Answer from the drawing. Dimensions are ordinates in mm from the lowest x, y and z of the part. A direction names the side the tool comes from. Round coordinates to 2 decimals unless told otherwise and drop trailing zeros. Write each loop counter-clockwise with the first axis right and the second up, starting at its lowest first coordinate (ties: lowest second). Pieces come first, ordered by that corner, then holes. Notation, with made-up numbers: (18, 69) -> (67, 69) arc R15 ccw to (67, 81) -> close; hole circle Ø7 at (-14, 81). An arc over 180 degrees is marked (long way). Return JSON: item names as keys, results as strings. Group by question number.
(1) For the marked faces 4 and 5, determine the directions among +Z, -Z, +X, -X, +Y, -Y from which every point of the face is accessible in a straight line to the end or side of a thin tool.
(2) Given pin 1 (2 mm diameter, centred on y = 4, z = 8.5, fed in from +X) (3 decimals); pin 2 (4 mm diameter, centred on x = 3.5, z = 8.5, fed in from +Y); pin 3 (1 mm diameter, centred on x = 3, z = 17.5, fed in from -Y), each flat-ended and moving along its own axis, determine where each tip first touches the part or whether it passes through.
(3) The mould has two halves that part along X. Classify the marked faces 1, 2 and 3: released by +X, released by -X, zero draft, split by the parting line, or undercut.
(4) A cutting plane is placed at D-D on z = 16.75. Give the vertices of the cut face in (x, y).
(5) A cutting plane is placed at B-B on y = 6.35. Give the vertices of the cut face in (x, z) (3 decimals).
(6) A cutting plane is placed at A-A on x = 6.35. Give the vertices of the cut face in (y, z) (3 decimals).
(7) A cutting plane is placed at C-C on x = 8.25. Give the vertices of the cut face in (y, z) (1 decimal).
(8) Straight lines are drawn through the part: line 1 (Y direction, x = 6.5, z = 9); line 2 (X direction, y = 1.5, z = 2.75). For each, find the intervals that lie inside material, in ascending order.
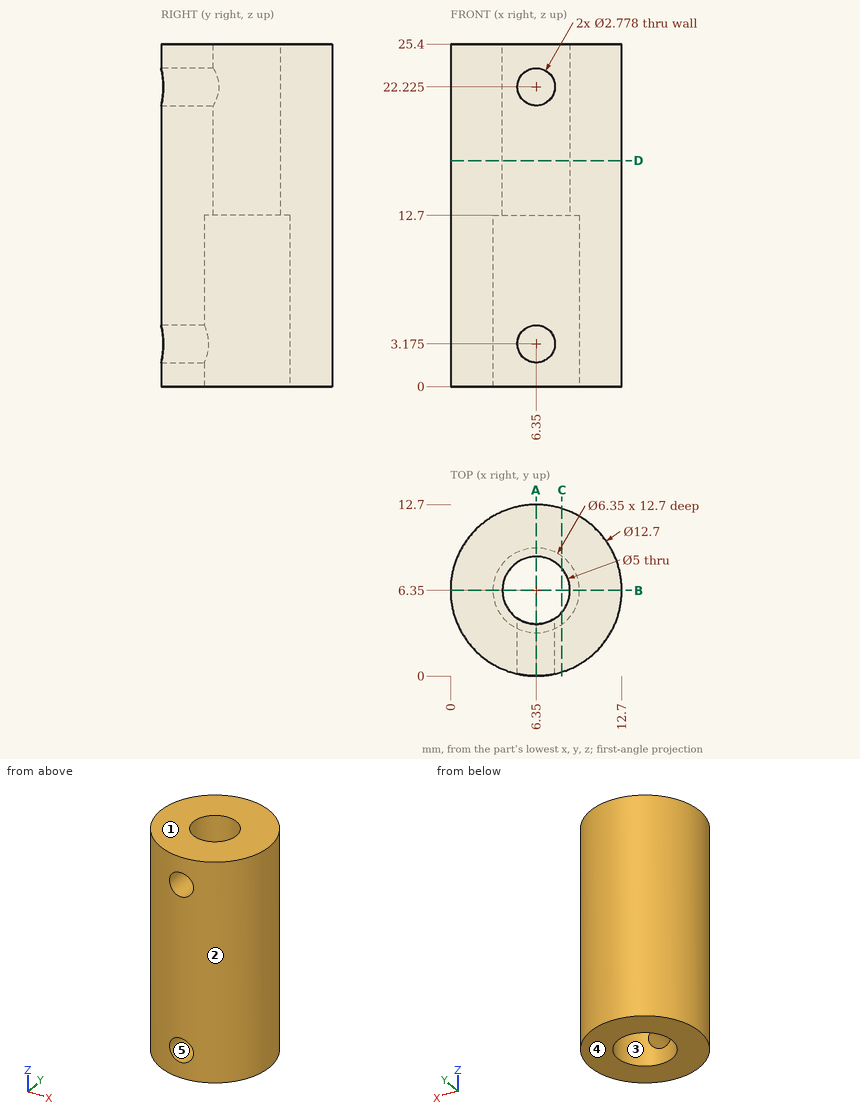
Checks:
{
 "1": {"face 4": "-Z, +X, -X, +Y, -Y", "face 5": "-Y"},
 "2": {"pin 1": "stops at x = 12.555", "pin 2": "stops at y = 12.64", "pin 3": "stops at y = 0.68"},
 "3": {"face 1": "zero draft", "face 2": "split by the parting line", "face 3": "undercut"},
 "4": {"outline": "circle Ø12.7 at (6.35, 6.35); hole circle Ø5 at (6.35, 6.35)"},
 "5": {"outline": "(0, 0) -> (3.175, 0) -> (3.175, 12.7) -> (3.85, 12.7) -> (3.85, 25.4) -> (0, 25.4) -> close; (8.85, 12.7) -> (9.525, 12.7) -> (9.525, 0) -> (12.7, 0) -> (12.7, 25.4) -> (8.85, 25.4) -> close"},
 "6": {"outline": "(0, 0) -> (3.175, 0) -> (3.175, 1.786) -> (0, 1.786) -> close; (0, 4.564) -> (3.175, 4.564) -> (3.175, 12.7) -> (3.85, 12.7) -> (3.85, 20.836) -> (0, 20.836) -> close; (0, 23.614) -> (3.85, 23.614) -> (3.85, 25.4) -> (0, 25.4) -> close; (8.85, 12.7) -> (9.525, 12.7) -> (9.525, 0) -> (12.7, 0) -> (12.7, 25.4) -> (8.85, 25.4) -> close"},
 "7": {"outline": "(0.3, 0) -> (3.8, 0) -> (3.8, 12.7) -> (4.7, 12.7) -> (4.7, 25.4) -> (0.3, 25.4) -> close; (8, 12.7) -> (8.9, 12.7) -> (8.9, 0) -> (12.4, 0) -> (12.4, 25.4) -> (8, 25.4) -> close"},
 "8": {"line 1": "y = 0 to 3.18, 9.52 to 12.7", "line 2": "x = 2.25 to 5.03, 7.67 to 10.45"}
}
